from build123d import *

# Parameters (mm, degrees)
SKETCH1_R               = 38
BOSS_EXTRUDE1_DEPTH     = 0.3
CUT_EXTRUDE1_DEPTH      = 54.740952727
CUT_EXTRUDE1_DEPTH_BACK = 54.740952727
SKETCH2_R               = 1.015
FILLET2_R               = 0.5


with BuildPart() as part:
    # Sketch1 → Boss-Extrude1 (new body)
    with BuildSketch(Plane(origin=(0, 0, 0), x_dir=(1, 0, 0), z_dir=(0, 1, 0))):
        with Locations(Location((0, 0, 0), (0, 0, 270))):
            Circle(SKETCH1_R)
    extrude(amount=BOSS_EXTRUDE1_DEPTH)

    # Sketch2 → Cut-Extrude1 (cut, two sides: drawn at the far end of the back side and taken through both)
    with BuildSketch(Plane(origin=(0, 0.3, 0), x_dir=(1, 0, 0), z_dir=(0, 1, 0)).offset(-CUT_EXTRUDE1_DEPTH_BACK)):
        with BuildLine():
            ThreePointArc((-37.053075912, -1.865359337), (-37.012379228, -2.548290386), (-36.959096408, -3.230354883))
            ThreePointArc((-36.959096408, -3.230354883), (-34.955040212, -4.912246307), (-33.273148788, -2.908190111))
            ThreePointArc((-33.273148788, -2.908190111), (-33.321117688, -2.294148218), (-33.357755673, -1.679326196))
            ThreePointArc((-33.357755673, -1.679326196), (-35.298432363, 0.075317353), (-37.053075912, -1.865359337))
        make_face()
        with BuildLine():
            ThreePointArc((-16.911089383, -33.021584697), (-16.299305403, -33.327805859), (-15.681978812, -33.622693832))
            ThreePointArc((-15.681978812, -33.622693832), (-13.223390014, -32.728075967), (-14.118007879, -30.26948717))
            ThreePointArc((-14.118007879, -30.26948717), (-14.673768207, -30.004008509), (-15.22453869, -29.728326924))
            ThreePointArc((-15.22453869, -29.728326924), (-17.714442923, -30.531680464), (-16.911089383, -33.021584697))
        make_face()
        with Locations(Location((-9.752534436, -33.874039795, 0), (0, 0, 270))):
            Circle(SKETCH2_R)
        with BuildLine():
            ThreePointArc((20.141986529, -31.15622536), (20.713073824, -30.779515473), (21.277117596, -30.392338949))
            ThreePointArc((21.277117596, -30.392338949), (21.731650198, -27.81582966), (19.155140909, -27.361297059))
            ThreePointArc((19.155140909, -27.361297059), (18.647349481, -27.709860291), (18.133216983, -28.049000728))
            ThreePointArc((18.133216983, -28.049000728), (17.58398944, -30.606997817), (20.141986529, -31.15622536))
        make_face()
        with BuildLine():
            ThreePointArc((37.053075912, 1.865359337), (37.012379228, 2.548290386), (36.959096408, 3.230354883))
            ThreePointArc((36.959096408, 3.230354883), (34.955040212, 4.912246307), (33.273148788, 2.908190111))
            ThreePointArc((33.273148788, 2.908190111), (33.321117688, 2.294148218), (33.357755673, 1.679326196))
            ThreePointArc((33.357755673, 1.679326196), (35.298432363, -0.075317353), (37.053075912, 1.865359337))
        make_face()
        with BuildLine():
            ThreePointArc((16.911089383, 33.021584697), (16.299305403, 33.327805859), (15.681978812, 33.622693832))
            ThreePointArc((15.681978812, 33.622693832), (13.223390014, 32.728075967), (14.118007879, 30.26948717))
            ThreePointArc((14.118007879, 30.26948717), (14.673768207, 30.004008509), (15.22453869, 29.728326924))
            ThreePointArc((15.22453869, 29.728326924), (17.714442923, 30.531680464), (16.911089383, 33.021584697))
        make_face()
        with BuildLine():
            ThreePointArc((-20.141986529, 31.15622536), (-20.713073824, 30.779515473), (-21.277117596, 30.392338949))
            ThreePointArc((-21.277117596, 30.392338949), (-21.731650198, 27.81582966), (-19.155140909, 27.361297059))
            ThreePointArc((-19.155140909, 27.361297059), (-18.647349481, 27.709860291), (-18.133216983, 28.049000728))
            ThreePointArc((-18.133216983, 28.049000728), (-17.58398944, 30.606997817), (-20.141986529, 31.15622536))
        make_face()
        with BuildLine():
            Line((-29.015113588, 18.848957093), (-30.189135525, 19.611631658))
            ThreePointArc((-30.189135525, 19.611631658), (-33.493010206, 13.199176768), (-35.452120741, 6.256767133))
            Line((-35.452120741, 6.256767133), (-32.251582063, 5.6919201))
            ThreePointArc((-32.251582063, 5.6919201), (-27.833314361, -17.258885007), (-9.23942383, -31.41966816))
            add(Edge.make_bspline(
                [(-4.046231948, -31.037364692), (-6.510871152, -30.608176232), (-6.812515045, -32.026230627), (-9.23942383, -31.41966816)],
                knots=[0, 0, 0, 0, 1, 1, 1, 1], degree=3))
            ThreePointArc((-4.046231948, -31.037364692), (2.745296544, -31.179373741), (9.407517011, -29.852782512))
            Line((9.407517011, -29.852782512), (10.399363852, -33.000200476))
            ThreePointArc((10.399363852, -33.000200476), (4.361224586, -34.324039974), (-1.816118884, -34.552304007))
            Line((-1.816118884, -34.552304007), (-1.889603463, -35.950374111))
            ThreePointArc((-1.889603463, -35.950374111), (5.315682713, -35.605386071), (12.307541088, -33.830820746))
            Line((12.307541088, -33.830820746), (11.196443628, -30.776649429))
            ThreePointArc((11.196443628, -30.776649429), (28.863290038, -15.474914804), (31.82994272, 7.708258327))
            add(Edge.make_bspline(
                [(28.902262264, 12.014542689), (29.762893756, 9.665508298), (31.141786833, 10.113304221), (31.82994272, 7.708258327)],
                knots=[0, 0, 0, 0, 1, 1, 1, 1], degree=3))
            ThreePointArc((28.902262264, 12.014542689), (25.629481462, 17.967183419), (21.149509523, 23.073539974))
            Line((21.149509523, 23.073539974), (23.379330016, 25.506213517))
            ThreePointArc((23.379330016, 25.506213517), (27.544878285, 20.93895127), (30.831232471, 15.703346914))
            Line((30.831232471, 15.703346914), (32.078738987, 16.338742454))
            ThreePointArc((32.078738987, 16.338742454), (28.177327493, 22.406209304), (23.144579654, 27.574053613))
            Line((23.144579654, 27.574053613), (21.055138435, 25.084729329))
            ThreePointArc((21.055138435, 25.084729329), (-1.029975677, 32.733799812), (-22.59051889, 23.711409833))
            add(Edge.make_bspline(
                [(-24.856030316, 19.022822003), (-23.252022604, 20.942667934), (-24.329271788, 21.912926407), (-22.59051889, 23.711409833)],
                knots=[0, 0, 0, 0, 1, 1, 1, 1], degree=3))
            ThreePointArc((-24.856030316, 19.022822003), (-28.374778006, 13.212190322), (-30.557026534, 6.779242538))
            Line((-30.557026534, 6.779242538), (-33.778693868, 7.493986959))
            ThreePointArc((-33.778693868, 7.493986959), (-31.906102871, 13.385088704), (-29.015113588, 18.848957093))
        make_face()
        with BuildLine():
            Line((36.454916606, 10.725626099), (34.146703694, 9.912246307))
            ThreePointArc((34.146703694, 9.912246307), (31.595686664, 11.133848581), (32.817288938, 13.68486561))
            Line((32.817288938, 13.68486561), (35.12550185, 14.498245403))
            ThreePointArc((35.12550185, 14.498245403), (35.83988338, 12.629440181), (36.454916606, 10.725626099))
        make_face()
        with BuildLine():
            ThreePointArc((10.799774466, 33.806672736), (10.098368991, 35.07524688), (8.829794847, 34.373841405))
            Line((8.829794847, 34.373841405), (8.705294407, 33.941406855))
            ThreePointArc((8.705294407, 33.941406855), (9.406699882, 32.672832711), (10.675274026, 33.374238186))
            Line((10.675274026, 33.374238186), (10.799774466, 33.806672736))
        make_face()
    extrude(amount=CUT_EXTRUDE1_DEPTH + CUT_EXTRUDE1_DEPTH_BACK, mode=Mode.SUBTRACT)

    # Fillet2
    fillet2_edges = [part.edges().sort_by_distance(p)[0] for p in [
        (-9.23942383, 0.15, 31.41966816),
        (-35.452120741, 0.15, -6.256767133),
        (-30.189135525, 0.15, -19.611631658),
        (-29.015113588, 0.15, -18.848957093),
        (-33.778693868, 0.15, -7.493986959),
        (-30.557026534, 0.15, -6.779242538),
        (-24.856030316, 0.15, -19.022822003),
        (-22.59051889, 0.15, -23.711409833),
        (21.055138435, 0.15, -25.084729329),
        (23.144579654, 0.15, -27.574053613),
        (32.078738987, 0.15, -16.338742454),
        (30.831232471, 0.15, -15.703346914),
        (23.379330016, 0.15, -25.506213517),
        (21.149509523, 0.15, -23.073539974),
        (28.902262264, 0.15, -12.014542689),
        (31.82994272, 0.15, -7.708258327),
        (11.196443628, 0.15, 30.776649429),
        (12.307541088, 0.15, 33.830820746),
        (-1.889603463, 0.15, 35.950374111),
        (-1.816118884, 0.15, 34.552304007),
        (10.399363852, 0.15, 33.000200476),
        (9.407517011, 0.15, 29.852782512),
        (-4.046231948, 0.15, 31.037364692),
        (-32.251582063, 0.15, -5.6919201),
    ]]
    fillet(fillet2_edges, radius=FILLET2_R)


solid = part.part
Part model, mm, in its own coordinate system. Give positions to 0.01 mm unless a question says otherwise; leave off trailing zeros. Order: outer loops, then holes, each group sorted by start corner. A loop starts at its lowest first (then second) coordinate and runs counter-clockwise, first axis right, second up. Notation, with made-up numbers: (0.5, 81) - (43.5, 81) arc R14 ccw to (43.5, 98) - close; hole circle Ø9 at (2, 87.25). An arc over 180 degrees is marked (long way). Use a Markdown table: item, result.
1) Two-plate mould, pull along Z, no slides. Class faces 1 (the cylindrical face through (-9.71, 0.15, 32.86)), 2 (the flat face through (23, 0.3, -23)), 3 (the cylindrical face through (25.82, 0.15, -17.69)): +Z half, -Z half, draft (parallel to the pull), parting line (faces both ways), or undercut.
Checked values:
| item | result |
|---|---|
| face 1 | undercut |
| face 2 | draft |
| face 3 | undercut |
2) Saw through at C-C on y = 0.15. Count the separate pieces of the cut face and the enclosed holes in it, plus the area to 3 significant figures.
Checked values:
| item | result |
|---|---|
| separate pieces | 1 |
| enclosed holes | 9 |
| area | 1,050 mm² |
3) Saw through at A-A on x = 0. List the corners of the cut face in (y, z).
Checked values:
| item | result |
|---|---|
| outline | (0, -38) - (0.3, -38) - (0.3, -32.75) - (0, -32.75) - close; (0, 31.3) - (0.3, 31.3) - (0.3, 34.6) - (0, 34.6) - close; (0, 36) - (0.3, 36) - (0.3, 38) - (0, 38) - close |
4) Probe L1, parallel to X at y = 0.2, z = 2.5; L2, parallel to Z at x = 10.5, y = 0.2; L3, parallel to X at y = 0.2, z = -24. List the from-to ranges inside material, lowest first. Write a range as from..to.
Checked values:
| item | result |
|---|---|
| L1 | -37.92..-37.02, -33.31..-32.65, 32.65..37.92 |
| L2 | -36.52..-34.85, -33.03..-31.02, 34.43..36.52 |
| L3 | -29.46..-22.28, 22..24.92, 26.83..29.46 |
5) Saw through at B-B on z = 13. List the corners of the cut face in (x, y).
Checked values:
| item | result |
|---|---|
| outline | (-35.71, 0) - (-30.06, 0) - (-30.06, 0.3) - (-35.71, 0.3) - close; (30.06, 0) - (35.71, 0) - (35.71, 0.3) - (30.06, 0.3) - close |
6) Saw through at D-D on x = 28. List the corners of the cut face in (y, z).
Checked values:
| item | result |
|---|---|
| outline | (0, -25.69) - (0.3, -25.69) - (0.3, -22.63) - (0, -22.63) - close; (0, -20.33) - (0.3, -20.33) - (0.3, -13.99) - (0, -13.99) - close; (0, 16.99) - (0.3, 16.99) - (0.3, 25.69) - (0, 25.69) - close |
